The listing builds one solid part. Answer for the finished solid, in the listing's coordinates (mm). Coordinates: 2 decimals unless noted, no trailing zeros. Write each loop counter-clockwise with the first axis right and the second up, starting at its lowest first coordinate (ties: lowest second). Pieces come first, ordered by that corner, then holes. Notation, with made-up numbers: M -22.75,13.25 L 4.25,13.25 A18 cw 4.25,44.25 Z; hole C 11.5,59 d2. An arc over 180 degrees is marked long. Put each result on its own line as item: value. Start each with the question number.
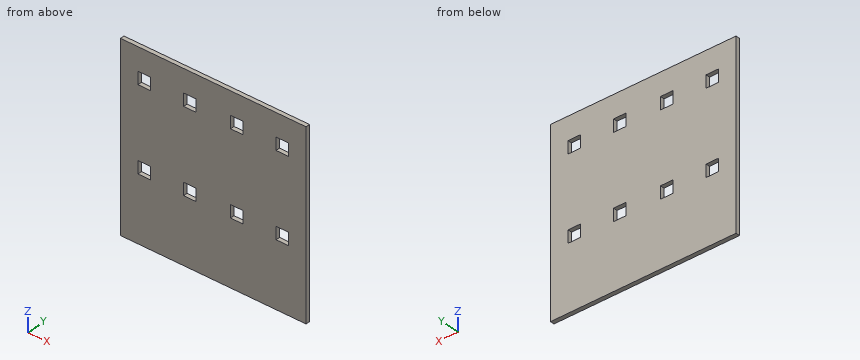
Autodesk Fusion 360 part; units mm, degrees
sketch "Sketch1" plane through (0, 0, 0) normal (0, 1, 0) x (1, 0, 0)
  line L0 (0, 0) -> (270, 0)
  line L1 (270, 0) -> (270, -264)
  line L2 (270, -264) -> (0, -264)
  line L3 (0, -264) -> (0, 0)
  dimension "d1" = 270
  dimension "d2" = 264
extrude "Extrude1" add sketch "Sketch1" along normal blind 6
sketch "Sketch2" plane through (0, 0, 0) normal (0, -1, 0) x (1, 0, 0)
  line L0 (270, 264) -> (0, 264)
  line L1 (0, 264) -> (0, 0)
  line L2 (0, 0) -> (270, 0)
  line L3 (270, 0) -> (270, 264)
  line L4 (25.625, 231.1665) -> (43.625, 231.1665)
  line L5 (43.625, 231.1665) -> (43.625, 213.1665)
  line L6 (43.625, 213.1665) -> (25.625, 213.1665)
  line L7 (25.625, 213.1665) -> (25.625, 231.1665)
  line L8 (91.875, 231.1665) -> (109.875, 231.1665)
  line L9 (109.875, 231.1665) -> (109.875, 213.1665)
  line L10 (109.875, 213.1665) -> (91.875, 213.1665)
  line L11 (91.875, 213.1665) -> (91.875, 231.1665)
  line L12 (160.125, 231.1665) -> (178.125, 231.1665)
  line L13 (178.125, 231.1665) -> (178.125, 213.1665)
  line L14 (178.125, 213.1665) -> (160.125, 213.1665)
  line L15 (160.125, 213.1665) -> (160.125, 231.1665)
  line L16 (226.375, 231.1665) -> (244.375, 231.1665)
  line L17 (244.375, 231.1665) -> (244.375, 213.1665)
  line L18 (244.375, 213.1665) -> (226.375, 213.1665)
  line L19 (226.375, 213.1665) -> (226.375, 231.1665)
  line L20 (25.625, 111.6665) -> (43.625, 111.6665)
  line L21 (43.625, 111.6665) -> (43.625, 93.6665)
  line L22 (43.625, 93.6665) -> (25.625, 93.6665)
  line L23 (25.625, 93.6665) -> (25.625, 111.6665)
  line L24 (91.875, 111.6665) -> (109.875, 111.6665)
  line L25 (109.875, 111.6665) -> (109.875, 93.6665)
  line L26 (109.875, 93.6665) -> (91.875, 93.6665)
  line L27 (91.875, 93.6665) -> (91.875, 111.6665)
  line L28 (160.125, 111.6665) -> (178.125, 111.6665)
  line L29 (178.125, 111.6665) -> (178.125, 93.6665)
  line L30 (178.125, 93.6665) -> (160.125, 93.6665)
  line L31 (160.125, 93.6665) -> (160.125, 111.6665)
  line L32 (226.375, 111.6665) -> (244.375, 111.6665)
  line L33 (244.375, 111.6665) -> (244.375, 93.6665)
  line L34 (244.375, 93.6665) -> (226.375, 93.6665)
  line L35 (226.375, 93.6665) -> (226.375, 111.6665)
  dimension "d5" = 18
  dimension "d6" = 18
  dimension "d7" = 18
  dimension "d8" = 18
  dimension "d9" = 18
  dimension "d10" = 18
  dimension "d11" = 270
  dimension "d12" = 264
  dimension "d13" = 25.625
  dimension "d17" = 32.8335
  dimension "d18" = 152.3335
  dimension "d19" = 48.25
  dimension "d22" = 48.25
  dimension "d24" = 25.625
extrude "Extrude2" cut sketch "Sketch2" against normal blind 6 contours L4 L5 L6 L7 | L8 L9 L10 L11 | L12 L13 L14 L15 | L16 L17 L18 L19 | L20 L21 L22 L23 | L24 L25 L26 L27 | L28 L29 L30 L31 | L32 L33 L34 L35
equation "d13 = 3 mm + ( ( 63.25 / 2 ) * 1 mm ) - ( ( 18 / 2 ) * 1 mm )"
equation "d17 = 3 mm + ( ( 77.667 / 2 ) * 1 mm ) - ( ( 18 / 2 ) * 1 mm )"
equation "d18 = 122.5 mm + ( ( 77.667 / 2 ) * 1 mm ) - ( ( 18 / 2 ) * 1 mm )"
equation "d19 = 3 mm + 63.25 mm - 18 mm"
equation "d22 = 3 mm + 63.25 mm - 18 mm"
equation "d24 = 3 mm + ( ( 63.25 / 2 ) * 1 mm ) - ( ( 18 / 2 ) * 1 mm )"
1) A cutting plane is placed at A-A on z = 99.5. Write down the section's boundary in (x, y) (3 decimals).
2) A cutting plane is placed at C-C on y = 3. State how many separate pieces and enclosed holes the cut face has, then the cut area to 3 significant figures.
3) A cutting plane is placed at B-B on x = 230.5. Write down the section's boundary in (y, z), then the cut area to 3 significant figures.
4) Straight lines are drawn through the part: probe 1 along Z at (x, y) = (102.5, 0.7); probe 2 along X at (y, z) = (3.1, 230) (3 decimals). For each, find the intervals that lie inside material, in ascending order.
Answers follow:
1. outline: M 0,0 L 25.625,0 L 25.625,6 L 0,6 Z; M 43.625,0 L 91.875,0 L 91.875,6 L 43.625,6 Z; M 109.875,0 L 160.125,0 L 160.125,6 L 109.875,6 Z; M 178.125,0 L 226.375,0 L 226.375,6 L 178.125,6 Z; M 244.375,0 L 270,0 L 270,6 L 244.375,6 Z
2. separate pieces: 1
2. enclosed holes: 8
2. area: 68,700 mm²
3. outline: M 0,0 L 6,0 L 6,93.67 L 0,93.67 Z; M 0,111.67 L 6,111.67 L 6,213.17 L 0,213.17 Z; M 0,231.17 L 6,231.17 L 6,264 L 0,264 Z
3. area: 1,370 mm²
4. probe 1: z = 0 to 93.67, 111.67 to 213.17, 231.17 to 264
4. probe 2: x = 0 to 25.625, 43.625 to 91.875, 109.875 to 160.125, 178.125 to 226.375, 244.375 to 270
